Autodesk Inventor part; units mm, degrees
ref_plane "YZ Plane" through (0, 0, 0) normal (1, 0, 0) x (0, 1, 0)
ref_plane "XY Plane" through (0, 0, 0) normal (0, 0, 1) x (1, 0, 0)
sketch "Эскиз1" plane through (0, 0, 0) normal (0, 1, 0) x (-1, 0, 0)
  circle A0 centre (0, 0) radius 40
  line L0 (40, 0) -> (0, -40)
  line L1 (0, -40) -> (-40, 0)
  line L2 (-40, 0) -> (0, 40)
  line L3 (0, 40) -> (40, 0)
  dimension "d0" = 80
ref_plane "РабПлоскость1" through (0, 90, 0) normal (0, 1, 0) x (-1, 0, 0)
sketch "Эскиз2" plane through (0, 90, 0) normal (0, 1, 0) x (-1, 0, 0)
  point P0 (0, 0)
  point P1 (0, 0)
loft "Лофт1" add profiles "Эскиз1" section 1 point at (0, 90, 0) contours L0 L1 L2 L3
sketch "Эскиз3" plane through (0, 0, 0) normal (0, 0, 1) x (1, 0, 0)
  line L0 (0, 0) -> (0, 10)
  line L1 (0, 90) -> (0, 0)
  line L2 (0, 10) -> (10, 10)
  line L3 (10, 10) -> (10, 44)
  line L4 (10, 44) -> (-10, 44)
  line L5 (0, 10) -> (-25, 10)
  line L6 (-25, 10) -> (-10, 44)
extrude "Выдавливание1" cut sketch "Эскиз3" against normal mid plane 90
Can you work these out from the model? Positions are in its coordinate system, mm. A direction names the side the tool comes from. Coordinates: 2 decimals unless noted, no trailing zeros. Loops run counter-clockwise (first coordinate to the right, second up) from the corner with the lowest first, then second, coordinate; pieces in that order, holes last. Notation, with made-up numbers: M 81,51 L 88,51 A23 ccw 88,76 Z; hole C 86,-31.5 d8. An arc over 180 degrees is marked long. Answer as CSV lines item,"result". Start each with the question number.
1. Suppose I cut it at C-C, the plane y = 29. List the corners of the cut face in (x, z) for me, plus the area to 3 significant figures.
2. If I drill on probe 1 along X at (y, z) = (29.5, 2); probe 2 along X at (y, z) = (27, -2); probe 3 along Y at (x, z) = (7, -26), over which ranges is the centre line in solid material (lowest first)? Write a range as [from, to].
3. Thinking about a two-plate mould opening in X: for faces 3 (the face through (-1, 0, -1)), 4 (the face through (-16.07, 31.46, 9.95)), 5 (the face through (-17.605, 26.762, 0.148)), which applies, +X half, -X half, draft (parallel to the pull), parting line (faces both ways), or undercut?
4. For pin 1 Ø4 at (x, z) = (-8.5, 29) entering from +Y; pin 2 Ø6 at (x, z) = (2, -0.5) entering from -Y; pin 3 Ø1 at (y, z) = (16, 3) entering from +X; pin 4 Ø1.5 at (x, y) = (-25, 19.5) entering from -Z, each with a flat end and sliding along its axis, tell me the tip position at first contact or that it passes through.
5. Suppose I cut it at B-B, the plane x = -7.5. List the corners of the cut face in (y, z) for me (3 decimals).
6. Suppose I cut it at D-D, the plane z = 17.5. List the corners of the cut face in (x, y) for me (3 decimals), plus the area to 3 significant figures.
7. For faces 1 (the face through (-15.9, 31.5, -10.1)), 2 (the face through (10, 23, 0)), which set-ups out of +Z, -Z, +X, -X, +Y, -Y let a thin tool reach every point of the face, with its end or its side?
8. Suppose I cut it at A-A, the plane z = 5. List the corners of the cut face in (x, y) for me.
Output:
1,outline,"M -27.11,0 L -16.62,-10.49 L -16.62,10.49 Z; M 10,-17.11 L 27.11,0 L 10,17.11 Z"
1,area,"403 mm^2"
2,probe 1,"x = [-24.89, -16.4], [10, 24.89]"
2,probe 2,"x = [-26, -17.5], [10, 26]"
2,probe 3,"y = [0, 10]"
3,face 3,"draft"
3,face 4,"-X half"
3,face 5,"undercut"
4,pin 1,"stops at y = 10"
4,pin 2,"stops at y = 0"
4,pin 3,"stops at x = 30.44"
4,pin 4,"stops at z = -7.15"
5,outline,"M 0,-32.5 L 10,-28.056 L 10,28.056 L 0,32.5 Z; M 44,-12.944 L 73.125,0 L 44,12.944 Z"
6,outline,"M -22.5,0 L 22.5,0 L 10,28.125 L 10,10 L -18.056,10 Z; M -2.944,44 L 2.944,44 L 0,50.625 Z"
6,area,"498 mm^2"
7,face 1,"-Z, -X, +Y"
7,face 2,"+Z, -Z"
8,outline,"M -35,0 L 35,0 L 0,78.75 Z; hole M -25,10 L 10,10 L 10,44 L -10,44 Z"
